```python
from build123d import *

# Parameters (mm, degrees)
SKETCH_1_R      = 2.2499999999999964
SKETCH_1_R_2    = 3.5000000000000075
EXTRUDE_3_DEPTH = 3
EXTRUDE_START   = 3
SKETCH_1_9_R    = 3.5000000000000075
EXTRUDE_4_DEPTH = 10
EXTRUDE_START_2 = 13
EXTRUDE_5_DEPTH = 40
CHAMFER_1_SIZE  = 20


with BuildPart() as part:
    # 草图1 → 凸台-拉伸3 (new body)
    # profile 1 of 5: a face of its own
    with BuildSketch(Plane(origin=(0, 0, 0), x_dir=(1, 0, 0), z_dir=(0, 1, 0))):
        with BuildLine():
            Line((81.76337811025178, -25), (85.93747727272425, -25))
            ThreePointArc((85.93747727272427, -25.00000000000003), (89.47720115518152, 2.0200181769446033), (84.72170874814934, 28.85276532316719))
            ThreePointArc((84.72170874814934, 28.852765323167215), (77.54750127881047, 41.87005748540227), (80.9872265222124, 27.41020138999083))
            ThreePointArc((80.98722652221241, 27.41020138999082), (85.49062597438983, 1.266045223118958), (81.76337811025176, -25.00000000000003))
        make_face()
        with BuildLine():
            ThreePointArc((79.50393531376338, 31.454320365013906), (78.90792202113376, 38.10634440334943), (83.19867820645547, 32.988330432119156))
            ThreePointArc((83.19867820645547, 32.988330432119156), (82.49378450242521, 32.18772445937683), (81.58047617746915, 31.636622870612896))
            ThreePointArc((81.58047617746915, 31.636622870612896), (80.55609271252037, 31.387290279852397), (79.50393531376338, 31.454320365013903))
        make_face(mode=Mode.SUBTRACT)
    # profile 2 of 5: a face of its own
    with BuildSketch(Plane(origin=(0, 0, 0), x_dir=(1, 0, 0), z_dir=(0, 1, 0))):
        with BuildLine():
            ThreePointArc((83.19867820645547, 32.988330432119156), (78.90792202113373, 38.10634440334942), (79.50393531376338, 31.454320365013903))
            ThreePointArc((79.50393531376338, 31.454320365013903), (80.55609271252037, 31.387290279852397), (81.58047617746915, 31.636622870612896))
            ThreePointArc((81.58047617746915, 31.636622870612896), (82.49378450242521, 32.18772445937683), (83.19867820645547, 32.988330432119156))
        make_face()
        with Locations(Location((80.25, 34.873879910328284, 0), (0, 0, 270))):
            Circle(SKETCH_1_R, mode=Mode.SUBTRACT)
    # profile 3 of 5: a face of its own
    with BuildSketch(Plane(origin=(0, 0, 0), x_dir=(1, 0, 0), z_dir=(0, 1, 0))):
        with BuildLine():
            ThreePointArc((-84.72170874814935, 28.85276532316715), (-89.4772011551815, 2.020018176944596), (-85.93747727272427, -25.00000000000001))
            Line((-85.93747727272425, -25), (-81.76337811025178, -25))
            ThreePointArc((-81.76337811025176, -25.000000000000007), (-85.49062597438983, 1.2660452231190007), (-80.98722652221241, 27.41020138999083))
            ThreePointArc((-80.98722652221241, 27.41020138999083), (-77.54750127881069, 41.87005748540241), (-84.72170874814934, 28.852765323167137))
        make_face()
        with Locations((-80.25, 34.873879910328284)):
            Circle(SKETCH_1_R_2, mode=Mode.SUBTRACT)
    # profile 4 of 5: a face of its own
    with BuildSketch(Plane(origin=(0, 0, 0), x_dir=(1, 0, 0), z_dir=(0, 1, 0))):
        with Locations((-80.25, 34.873879910328284)):
            Circle(SKETCH_1_R_2)
        with Locations(Location((-80.25, 34.873879910328284, 0), (0, 0, 270))):
            Circle(SKETCH_1_R, mode=Mode.SUBTRACT)
    # profile 5 of 5: a face of its own
    with BuildSketch(Plane(origin=(0, 0, 0), x_dir=(1, 0, 0), z_dir=(0, 1, 0))):
        with BuildLine():
            Line((-81.76337811025178, -25), (-85.93747727272425, -25))
            ThreePointArc((-85.93747727272427, -25.00000000000001), (3.55e-15, -89.5), (85.93747727272427, -25.00000000000003))
            Line((85.93747727272425, -25), (81.76337811025178, -25))
            ThreePointArc((81.76337811025176, -25.00000000000003), (-3.55e-15, -85.5), (-81.76337811025176, -25.000000000000007))
        make_face()
    extrude(amount=EXTRUDE_3_DEPTH)

    # 草图1<9> → 凸台-拉伸4 (add)
    # profile 1 of 3: a face of its own
    with BuildSketch(Plane(origin=(0, 0, 0), x_dir=(1, 0, 0), z_dir=(0, 1, 0)).offset(EXTRUDE_START)):
        with BuildLine():
            ThreePointArc((-84.72170874814935, 28.85276532316715), (-89.4772011551815, 2.020018176944596), (-85.93747727272427, -25.00000000000001))
            Line((-85.93747727272425, -25), (-81.76337811025178, -25))
            ThreePointArc((-81.76337811025176, -25.000000000000007), (-85.49062597438983, 1.2660452231190007), (-80.98722652221241, 27.41020138999083))
            ThreePointArc((-80.98722652221241, 27.41020138999083), (-77.54750127881069, 41.87005748540241), (-84.72170874814934, 28.852765323167137))
        make_face()
        with Locations(Location((-80.25, 34.873879910328284, 0), (0, 0, 270))):
            Circle(SKETCH_1_9_R, mode=Mode.SUBTRACT)
    # profile 2 of 3: a face of its own
    with BuildSketch(Plane(origin=(0, 0, 0), x_dir=(1, 0, 0), z_dir=(0, 1, 0)).offset(EXTRUDE_START)):
        with BuildLine():
            Line((-81.76337811025178, -25), (-85.93747727272425, -25))
            ThreePointArc((-85.93747727272427, -25.00000000000001), (3.55e-15, -89.5), (85.93747727272427, -25.00000000000003))
            Line((85.93747727272425, -25), (81.76337811025178, -25))
            ThreePointArc((81.76337811025176, -25.00000000000003), (-3.55e-15, -85.5), (-81.76337811025176, -25.000000000000007))
        make_face()
    # profile 3 of 3: a face of its own
    with BuildSketch(Plane(origin=(0, 0, 0), x_dir=(1, 0, 0), z_dir=(0, 1, 0)).offset(EXTRUDE_START)):
        with BuildLine():
            Line((81.76337811025178, -25), (85.93747727272425, -25))
            ThreePointArc((85.93747727272427, -25.00000000000003), (89.47720115518152, 2.0200181769446033), (84.72170874814934, 28.85276532316719))
            ThreePointArc((84.72170874814934, 28.852765323167215), (77.54750127881047, 41.87005748540227), (80.9872265222124, 27.41020138999083))
            ThreePointArc((80.98722652221241, 27.41020138999082), (85.49062597438983, 1.266045223118958), (81.76337811025176, -25.00000000000003))
        make_face()
        with BuildLine():
            ThreePointArc((79.50393531376338, 31.454320365013906), (78.90792202113376, 38.10634440334943), (83.19867820645547, 32.988330432119156))
            ThreePointArc((83.19867820645547, 32.988330432119156), (82.49378450242521, 32.18772445937683), (81.58047617746915, 31.636622870612896))
            ThreePointArc((81.58047617746915, 31.636622870612896), (80.55609271252037, 31.387290279852397), (79.50393531376338, 31.454320365013903))
        make_face(mode=Mode.SUBTRACT)
    extrude(amount=EXTRUDE_4_DEPTH)

    # 草图1<10> → 凸台-拉伸5 (add)
    with BuildSketch(Plane(origin=(0, 0, 0), x_dir=(1, 0, 0), z_dir=(0, 1, 0)).offset(EXTRUDE_START_2)):
        with BuildLine():
            Line((-81.76337811025178, -25), (-85.93747727272425, -25))
            ThreePointArc((-85.93747727272427, -25.00000000000001), (3.55e-15, -89.5), (85.93747727272427, -25.00000000000003))
            Line((85.93747727272425, -25), (81.76337811025178, -25))
            ThreePointArc((81.76337811025176, -25.00000000000003), (-3.55e-15, -85.5), (-81.76337811025176, -25.000000000000007))
        make_face()
    extrude(amount=EXTRUDE_5_DEPTH)

    # 倒角1
    chamfer_1_edges = [part.edges().sort_by_distance(p)[0] for p in [
        (-83.85042769148802, 13, 25),
        (83.85042769148802, 13, 25),
    ]]
    chamfer(chamfer_1_edges, length=CHAMFER_1_SIZE)


solid = part.part
```
Geometry check sheet. Reference: the model listing, model coordinates, mm. A direction names the side the tool comes from. Give positions to 0.01 mm unless a question says otherwise; leave off trailing zeros. Write each loop counter-clockwise with the first axis right and the second up, starting at its lowest first coordinate (ties: lowest second). Pieces come first, ordered by that corner, then holes.
1) Gauge pin test, flat ends, axial feed: pin 1 (11 mm diameter, centred on x = 80.25, z = -34.87, fed in from -Y); pin 2 (1.5 mm diameter, centred on y = 16.5, z = 32.5, fed in from +X); pin 3 (6.5 mm diameter, centred on x = -80.25, z = -34.87, fed in from +Y); pin 4 (3.5 mm diameter, centred on x = -83.5, y = 46.5, fed in from -Z). Record the tip position at first contact, or that the pin passes through.
2) Release check for a two-part mould opening along Z. For faces 4 (the flat face through (-84, 13, -24)), 5 (the cylindrical face through (77.1, 7.9, -36.4)), 6 (the cylindrical face through (-81.59, 7.93, -31.64)), 7 (the flat face through (86, 23, 15)) record: pulls with the +Z half, pulls with the -Z half, needs draft (parallel to the pull), parting line crosses it, or undercut.
3) Access from +Z, -Z, +X, -X, +Y, -Y to the whole of each face (thin tool, end or side, straight path). Record for faces 1 (the flat face through (83, 13, -22)), 2 (the cylindrical face through (-77.269, 6.409, -41.756)), 3 (the flat face through (-78, 3, -34)).
4) Section check D-D, the plane x = 0. Record the boundary of the cut face in (y, z).
5) Material ranges on L1, parallel to X at y = 27, z = 25; L2, parallel to X at y = 36.5, z = 45.5; L3, parallel to Z at x = 2.5, y = 32, recorded low to high.
6) Section check C-C, the plane y = 38.5. Record the boundary of the cut face in (x, z), and give its area (3 significant figures).
7) Section check B-B, the plane z = 28.5. Record the boundary of the cut face in (x, y), and give its area (3 significant figures).
8) Section check A-A, the plane z = 0. Record the boundary of the cut face in (x, y).
Computed:
1. pin 1: stops at y = 0
1. pin 2: stops at x = 83.68
1. pin 3: stops at y = 3
1. pin 4: stops at z = 25
2. face 4: needs draft
2. face 5: undercut
2. face 6: undercut
2. face 7: pulls with the -Z half
3. face 1: -Z, +X, -X, +Y
3. face 2: +Y, -Y
3. face 3: +Y
4. outline: (0, 85.5) - (53, 85.5) - (53, 89.5) - (0, 89.5) - close
5. L1: x = -85.94 to -81.76, 81.76 to 85.94
5. L2: x = -77.07 to -72.39, 72.39 to 77.07
5. L3: z = 85.46 to 89.47
6. outline: (-85.94, 25) - (-81.76, 25) arc R85.5 cw to (81.76, 25) - (85.94, 25) arc R89.5 ccw to start
6. area: 897 mm2
7. outline: (-84.84, 0) - (-80.61, 0) - (-80.61, 53) - (-84.84, 53) - close; (80.61, 0) - (84.84, 0) - (84.84, 53) - (80.61, 53) - close
7. area: 448 mm2
8. outline: (-89.5, 0) - (-85.5, 0) - (-85.5, 13) - (-89.5, 13) - close; (85.5, 0) - (89.5, 0) - (89.5, 13) - (85.5, 13) - close
